Can you work these out from the model? Positions are in its coordinate system, mm. Face numbers are marked on the shaded views. A direction names the side the tool comes from. Coordinates: 2 decimals unless noted, no trailing zeros. One line per question, with ' | ' between items. Start each with the question number.
from build123d import *

# Parameters (mm, degrees)
EXTRUDE1_DEPTH = 4.064
SKETCH14_W     = 4.826
SKETCH14_H     = 5.445676263


# Read off the part's stored shape, not the designer's step: Cut-Revolve5
with BuildPart() as part:
    # Sketch1 → Revolve1 (revolve)
    with BuildSketch(Plane.XY):
        Polygon((0, 0), (0, 7.161072654), (0.025429996, 7.208479528), (0.64160868, 8.357166473), (0.695379235, 8.358846887), (1.382081969, 7.25087702), (1.435852524, 7.252557434), (2.052031208, 8.401244379), (2.105801763, 8.402924793), (2.792504496, 7.294954927), (2.846275051, 7.296635341), (3.462453735, 8.445322286), (3.51622429, 8.4470027), (4.202927024, 7.339032834), (4.256697579, 7.340713248), (4.872876263, 8.489400193), (4.926646818, 8.491080606), (5.613349551, 7.38311074), (5.667120106, 7.384791154), (6.28329879, 8.533478099), (6.337069345, 8.535158513), (7.023772079, 7.427188647), (7.077542634, 7.428869061), (7.693721318, 8.577556006), (7.747491873, 8.57923642), (8.434194606, 7.471266554), (8.487965161, 7.472946968), (9.104143845, 8.621633913), (9.1579144, 8.623314326), (9.844617134, 7.51534446), (9.898387689, 7.517024874), (10.514566373, 8.665711819), (10.568336928, 8.667392233), (11.255039661, 7.559422367), (11.308810216, 7.561102781), (11.9249889, 8.709789726), (11.978759455, 8.71147014), (12.665462189, 7.603500274), (12.719232744, 7.605180687), (13.335411428, 8.753867633), (13.389181983, 8.755548046), (14.075884716, 7.64757818), (14.129655271, 7.649258594), (14.745833955, 8.797945539), (14.79960451, 8.799625953), (15.486307244, 7.691656087), (15.540077799, 7.693336501), (16.156256483, 8.842023446), (16.210027038, 8.84370386), (16.896729771, 7.735733994), (16.950500326, 7.737414407), (16.950500326, 0), align=None)
    revolve(axis=Axis((0, 0, 0), (-1, 0, 0)))

    # Sketch5 → Cut-Revolve2 (revolve, cut)
    with BuildSketch(Plane.XY, mode=Mode.PRIVATE) as cut_revolve2_sk:
        Polygon((12.192, 0), (12.192, 8.71813424), (16.950500326, 8.866844806), (16.950500326, 0), align=None)
    revolve(cut_revolve2_sk.sketch.rotate(Axis((0, 0, 0), (-1, 0, 0)), 180), axis=Axis((0, 0, 0), (-1, 0, 0)), mode=Mode.SUBTRACT)

    # Sketch7 → Extrude1 (add)
    with BuildSketch(Plane(origin=(12.192, 0, 0), x_dir=(0, 0, -1), z_dir=(1, 0, 0))):
        Polygon((-8.636, -4.985996925), (-8.636, 4.985996925), (0, 9.971993849), (8.636, 4.985996925), (8.636, -4.985996925), (0, -9.971993849), align=None)
    extrude(amount=EXTRUDE1_DEPTH)

    # Sketch10 → Cut-Revolve4 (revolve, cut)
    with BuildSketch(Plane.XY, mode=Mode.PRIVATE) as cut_revolve4_sk:
        Polygon((16.256, 9.971993849), (12.192, 9.971993849), (12.192, 8.066993849), (12.961873944, 9.717993849), (15.486126056, 9.717993849), (16.256, 8.066993849), align=None)
    revolve(cut_revolve4_sk.sketch.rotate(Axis((0, 0, 0), (1, 0, 0)), 297.29455937), axis=Axis((0, 0, 0), (1, 0, 0)), mode=Mode.SUBTRACT)

    # Cut-Revolve5 outline → Cut-Revolve5 (revolve, cut)
    with BuildSketch(Plane.YX):
        Polygon((0, 16.256), (0, 4.826), (5.445676263, 4.826), (6.661157266, 5.429898935), (6.664521379, 5.48366949), (5.578673669, 6.204558764), (5.582037782, 6.258329319), (6.749270061, 6.838256384), (6.752634175, 6.892026939), (5.666786464, 7.612916212), (5.670150578, 7.666686767), (6.837382857, 8.246613832), (6.84074697, 8.300384387), (5.75489926, 9.021273661), (5.758263373, 9.075044216), (6.925495653, 9.654971281), (6.928859766, 9.708741836), (5.843012056, 10.42963111), (5.846376169, 10.483401665), (7.013608448, 11.063328729), (7.016972562, 11.117099284), (5.931124851, 11.837988558), (5.934488965, 11.891759113), (7.101721244, 12.471686178), (7.105085357, 12.525456733), (6.019237647, 13.246346007), (6.02260176, 13.300116562), (7.18983404, 13.880043627), (7.193198153, 13.933814182), (6.107350443, 14.654703455), (6.110714556, 14.70847401), (7.277946835, 15.288401075), (7.281310949, 15.34217163), (6.195463238, 16.063060904), (6.198827352, 16.116831459), (6.478935012, 16.256), align=None)
    revolve(axis=Axis((0, 0, 0), (1, 0, 0)), mode=Mode.SUBTRACT)

    # Sketch14 → Cut-Revolve6 (revolve, cut)
    with BuildSketch(Plane.XY, mode=Mode.PRIVATE) as cut_revolve6_sk:
        with Locations((2.413, 2.722838132)):
            Rectangle(SKETCH14_W, SKETCH14_H)
    revolve(cut_revolve6_sk.sketch.rotate(Axis((0, 0, 0), (-1, 0, 0)), 180), axis=Axis((0, 0, 0), (-1, 0, 0)), mode=Mode.SUBTRACT)


solid = part.part
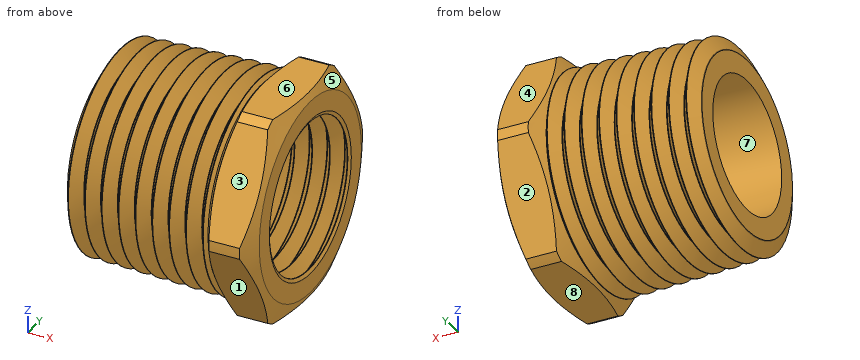
(1) If we mould it in two halves opening along Z, with no side actions, what happens to the marked faces 5, 6, 7 and 8? For each: +Z half, -Z half, draft (parallel to the pull), parting line (faces both ways), or undercut.
(2) I'm going to push flat-ended pins straight in: pin 1 (3 mm diameter, centred on x = 10.5, z = 3.5, fed in from -Y); pin 2 (4 mm diameter, centred on x = 11.5, y = -3, fed in from -Z); pin 3 (5 mm diameter, centred on x = 4.5, y = 1.5, fed in from +Z). Where does each tip first touch, or does it pass through?
(3) If I drill on probe 1 along Z at (x, y) = (1.35, 0); probe 2 along Z at (x, y) = (6, -4.25); probe 3 along Y at (x, z) = (2.75, 1), over which ranges is the centre line in solid material (lowest first)?
(4) Which directions (+Z, -Z, +X, -X, +Y, -Y) give clear straight access to the entire face, cutting with the end or side of a thin tool? Please do the marked faces 1, 2, 3 and 4.
Values:
1) face 5: parting line | face 6: +Z half | face 7: undercut | face 8: -Z half
2) pin 1: y = -8.43 | pin 2: z = -8.65 | pin 3: z = 8.54
3) probe 1: -7.3 to -5.45, 5.45 to 7.3 | probe 2: -6.78 to -4.07, 4.07 to 6.78 | probe 3: -7.3 to -5.35, 5.35 to 7.3
4) face 1: -Z, +X, -Y | face 2: -Z, +X, +Y | face 3: +Z, +X, -Y | face 4: +Z, +X, +Y
